Autodesk Inventor part; units mm, degrees
ref_plane "YZ Plane" through (0, 0, 0) normal (1, 0, 0) x (0, 1, 0)
ref_plane "XZ Plane" through (0, 0, 0) normal (0, 1, 0) x (-1, 0, 0)
ref_plane "XY Plane" through (0, 0, 0) normal (0, 0, 1) x (1, 0, 0)
sketch "Sketch1" plane through (0, 0, 0) normal (0, 0, 1) x (1, 0, 0)
  line L0 (-48.3526, 6.9347) -> (16.6474, 6.9347)
  line L1 (16.6474, 6.9347) -> (16.6474, -38.0653)
  line L2 (16.6474, -38.0653) -> (-48.3526, -38.0653)
  line L3 (-48.3526, -38.0653) -> (-48.3526, 6.9347)
  circle A0 centre (-35.3526, -6.0653) radius 10
  circle A1 centre (-22.3526, -25.0653) radius 10
  circle A2 centre (-9.3526, -6.0653) radius 10
  circle A3 centre (3.6474, -25.0653) radius 10
  circle A4 centre (-40.3526, -30.0653) radius 5
  circle A5 centre (8.6474, -1.0653) radius 5
  circle A6 centre (-40.3526, -20.0653) radius 3
  circle A7 centre (8.6474, -11.0653) radius 3
  circle A8 centre (-9.3526, -33.0653) radius 2.75
  circle A9 centre (-22.3526, 1.9347) radius 2.75
  dimension "d1" = 65
  dimension "d2" = 45
  dimension "d3" = 20
  dimension "d10" = 13
  dimension "d11" = 13
  dimension "d40" = 20
  dimension "d41" = 20
  dimension "d42" = 20
  dimension "d43" = 13
  dimension "d44" = 13
  dimension "d45" = 39
  dimension "d46" = 39
  dimension "d47" = 10
  dimension "d48" = 10
  dimension "d49" = 8
  dimension "d50" = 8
  dimension "d51" = 8
  dimension "d52" = 8
  dimension "d53" = 6
  dimension "d54" = 6
  dimension "d55" = 18
  dimension "d56" = 18
  dimension "d57" = 5.5
  dimension "d58" = 5.5
  dimension "d59" = 5
  dimension "d60" = 5
extrude "Extrusion1" add sketch "Sketch1" along normal blind 2
chamfer "Chamfer2" distance 2 angle 45 2 edges at (-48.3526, -38.0653, 1) (16.6474, -38.0653, 1)
equation "\"d10\" = d11"
equation "\"d40\" = d3"
equation "\"d41\" = d3"
equation "\"d42\" = d3"
equation "\"d43\" = d11"
equation "\"d44\" = d11"
properties part number "CNCM_ALU_First_sieve" material "Aluminum 6061"
Can you work these out from the model? Positions are in its coordinate system, mm. Round coordinates to 2 decimals unless told otherwise and drop trailing zeros. Loops run counter-clockwise (first coordinate to the right, second up) from the corner with the lowest first, then second, coordinate; pieces in that order, holes last. Notation, with made-up numbers: M 22,-39.5 L 42,-39.5 A16 ccw 42,-15.5 Z; hole C 24.5,-23 d7. An arc over 180 degrees is marked long. Answer as a JSON object with one key per item and string values. Group by question number.
Q1. Imagine slicing it at A-A, the plane x = -9. Please give me the cut outline in (y, z), then the cut area to 3 significant figures.
Q2. Imagine slicing it at D-D, the plane z = 0.75. Count the separate pieces of the cut face and the enclosed holes in it, then the cut area to 3 significant figures.
Q3. We'd pull the mould along Y, two halves only. Please class faces 1 (the flat face through (-15, -38.065, 1)), 2 (the flat face through (-16, -15, 0)), 3 (the cylindrical face through (7.997, -8.137, 0.986)), 4 (the cylindrical face through (-25.814, -9.069, 0.986)): +Y half, -Y half, draft (parallel to the pull), parting line (faces both ways), or undercut.
Q4. Imagine slicing it at C-C, the plane y = -29. Please give me the cut outline in (x, z), then the cut area to 3 significant figures.
Q5. Imagine slicing it at B-B, the plane x = 8.5. Please give me the cut outline in (y, z).
Q6. Please list where these lines run through material, in increasing order: L1, parallel to X at y = -25, z = 0.75; L2, parallel to Y at x = -37, z = 1.85; L3, parallel to Y at x = -9.5, z = 0.4.
Findings:
{
 "1": {"outline": "M -38.07,0 L -35.79,0 L -35.79,2 L -38.07,2 Z; M -30.34,0 L -16.06,0 L -16.06,2 L -30.34,2 Z; M 3.93,0 L 6.93,0 L 6.93,2 L 3.93,2 Z", "area": "39.1 mm2"},
 "2": {"separate pieces": "1", "enclosed holes": "10", "area": "1,400 mm2"},
 "3": {"face 1": "-Y half", "face 2": "draft", "face 3": "undercut", "face 4": "undercut"},
 "4": {"outline": "M -48.35,0 L -45.24,0 L -45.24,2 L -48.35,2 Z; M -35.47,0 L -31.55,0 L -31.55,2 L -35.47,2 Z; M -13.16,0 L -5.55,0 L -5.55,2 L -13.16,2 Z; M 12.84,0 L 16.65,0 L 16.65,2 L 12.84,2 Z", "area": "36.9 mm2"},
 "5": {"outline": "M -38.07,0 L -33.81,0 L -33.81,2 L -38.07,2 Z; M -16.32,0 L -14.06,0 L -14.06,2 L -16.32,2 Z; M -8.07,0 L -6.06,0 L -6.06,2 L -8.07,2 Z; M 3.93,0 L 6.93,0 L 6.93,2 L 3.93,2 Z"},
 "6": {"L1": "x = -48.35 to -32.35, -12.35 to -6.35, 13.65 to 16.65", "L2": "y = -38.07 to -33.77, -26.36 to -15.93, 3.8 to 6.93", "L3": "y = -38.07 to -35.81, -30.32 to -16.06, 3.93 to 6.93"}
}
